Work out the finished part from the listing and answer in its coordinate system (mm). Face numbers are marked on the shaded views. A direction names the side the tool comes from. Give positions to 0.01 mm unless a question says otherwise; leave off trailing zeros. Loops run counter-clockwise (first coordinate to the right, second up) from the corner with the lowest first, then second, coordinate; pieces in that order, holes last. Notation, with made-up numbers: (24.5, 89) - (74.5, 89) arc R29 cw to (74.5, 112) - close; hole circle Ø10 at (-39, -21.5). An arc over 180 degrees is marked (long way). Use CSV: the item, a comma, the result in double quotes.
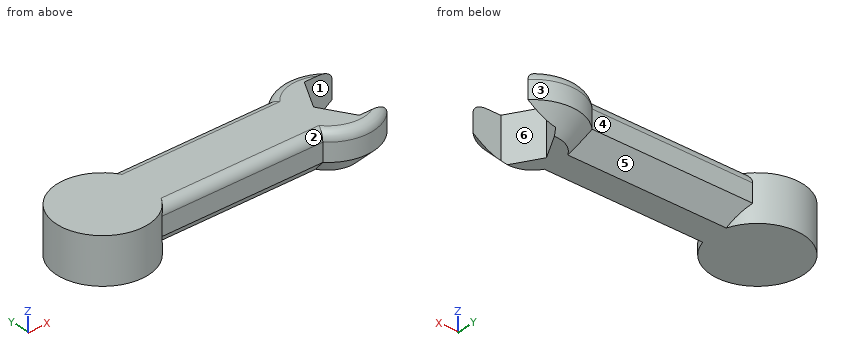
from build123d import *

# Parameters (mm, degrees)
F1_DEPTH = 6.35
F3_DEPTH = 12.701
F4_R     = 2.54
F5_SIZE  = 5.08


with BuildPart() as f1:
    # F0 (on Top) → F1 (new body, symmetric)
    with BuildSketch(Plane.XY):
        with BuildLine():
            Line((22.6803858958, 8.89), (-22.6803858958, 8.89))
            ThreePointArc((-22.6803858958, 8.89), (-44.45, 0), (-22.6803858958, -8.89))
            Line((-22.6803858958, -8.89), (22.6803858958, -8.89))
            ThreePointArc((22.6803858958, -8.89), (44.45, 0), (22.6803858958, 8.89))
        make_face()
    extrude(amount=F1_DEPTH, both=True)

    # F2 (on face) → F3 (cut, through all)
    with BuildSketch(Plane.XY.offset(6.35)):
        Polygon((27.8347122138, 0), (32.9673561069, -8.89), (43.2326438931, -8.89), (48.3652877862, 0), (43.2326438931, 8.89), (32.9673561069, 8.89), align=None)
    extrude(amount=-F3_DEPTH, mode=Mode.SUBTRACT)

    # F4
    f4_edges = [f1.edges().sort_by_distance(p)[0] for p in [
        (0, -8.89, 6.35),
        (31.75, -12.7, 6.35),
        (0, 8.89, 6.35),
        (31.75, 12.7, 6.35),
    ]]
    fillet(f4_edges, radius=F4_R)

    # F5
    f5_edges = [f1.edges().sort_by_distance(p)[0] for p in [
        (0, 8.89, -6.35),
        (31.75, 12.7, -6.35),
        (0, -8.89, -6.35),
        (31.75, -12.7, -6.35),
    ]]
    chamfer(f5_edges, length=F5_SIZE)


solid = f1.part
Item 1: The mould has two halves that part along Y. Classify the marked faces 1, 2 and 3: pulls with the +Y half, pulls with the -Y half, needs draft (parallel to the pull), parting line crosses it, or undercut.
Determined:
face 1,"undercut"
face 2,"pulls with the -Y half"
face 3,"pulls with the +Y half"
Item 2: A cutting plane is placed at C-C on y = -1.5. Determine the outline of the cut face in (x, z), and give its area (3 significant figures).
Determined:
outline,"(-44.36, -6.35) - (28.7, -6.35) - (28.7, 6.35) - (-44.36, 6.35) - close"
area,"928 mm²"
Item 3: For the marked faces 4, 5 and 6, determine the directions among +Z, -Z, +X, -X, +Y, -Y from which every point of the face is accessible in a straight line to the end or side of a thin tool.
Determined:
face 4,"+Z, -Z, +Y"
face 5,"-Z, +Y"
face 6,"+Z, -Z, +X"
Item 4: A cutting plane is placed at B-B on z = 3. Determine the outline of the cut face in (x, y).
Determined:
outline,"(-22.68, -8.89) - (22.68, -8.89) arc R12.7 ccw to (40.82, -8.89) - (32.97, -8.89) - (27.83, 0) - (32.97, 8.89) - (40.82, 8.89) arc R12.7 ccw to (22.68, 8.89) - (-22.68, 8.89) arc R12.7 ccw (long way) to start"
Item 5: Given P1, Ø1.5, axis at x = -4.5, z = 2.5, coming from the +Y side; P2, Ø2.5, axis at x = 37, z = 1.5, coming from the -Y side; P3, Ø4, axis at x = 38, z = 1, coming from the +Y side, each flat-ended and moving along its own axis, determine where each tip first touches the part or whether it passes through.
Determined:
P1,"stops at y = 8.89"
P2,"stops at y = -12.05"
P3,"stops at y = 11.97"
Item 6: A cutting plane is placed at D-D on z = -2.25. Determine the outline of the cut face in (x, y), and give its area (3 significant figures).
Determined:
outline,"(-21.81, -7.91) - (23.1, -7.91) arc R11.72 ccw to (39.39, -8.89) - (32.97, -8.89) - (27.83, 0) - (32.97, 8.89) - (39.39, 8.89) arc R11.72 ccw to (23.1, 7.91) - (-21.81, 7.91) arc R12.7 ccw (long way) to start"
area,"1,380 mm²"
Item 7: Find the intervals of material crossed by line 1 (Y direction, x = -20.5, z = -1); line 2 (Y direction, x = 30.5, z = 3); line 3 (X direction, y = -10, z = 2.5), in increasing order.
Determined:
line 1,"y = -8.89 to 8.89"
line 2,"y = -12.64 to -4.62, 4.62 to 12.64"
line 3,"x = -39.58 to -23.92, 23.92 to 39.58"
Item 8: A cutting plane is placed at A-A on x = -1. Determine the outline of the cut face in (y, z), and give its area (3 significant figures).
Determined:
outline,"(-8.89, -1.27) - (-3.81, -6.35) - (3.81, -6.35) - (8.89, -1.27) - (8.89, 3.81) arc R2.54 ccw to (6.35, 6.35) - (-6.35, 6.35) arc R2.54 ccw to (-8.89, 3.81) - close"
area,"197 mm²"
